from build123d import *

# Parameters (mm, degrees)
F1_DEPTH = 10.16


with BuildPart() as f1:
    # F0 (on Top) → F1 (new body)
    with BuildSketch(Plane.XY):
        with BuildLine():
            Line((-29.21, 0), (0, 0))
            Line((0, 0), (0, 8.128))
            Line((0, 8.128), (-6.604, 8.128))
            Line((-6.604, 8.128), (-6.604, 4.318))
            Line((-6.604, 4.318), (-7.62, 4.318))
            Line((-7.62, 4.318), (-7.62, 5.334))
            Line((-7.62, 5.334), (-7.62, 8.636))
            ThreePointArc((-7.62, 8.636), (-7.991974, 9.534026), (-8.89, 9.906))
            Line((-8.89, 9.906), (-26.67, 9.906))
            ThreePointArc((-26.67, 9.906), (-28.466051, 9.162051), (-29.21, 7.366))
            Line((-29.21, 7.366), (-29.21, 0))
        make_face()
    extrude(amount=F1_DEPTH)

    # F2: F1 across face


with BuildPart() as f1_1:
    add(f1.part)
    add(f1.part.mirror(Plane(origin=(0, 4.064, 5.08), x_dir=(0, 1, 0), z_dir=(1, 0, 0))))

    # F3: F1 across face


with BuildPart() as f1_2:
    add(f1_1.part)
    add(f1_1.part.mirror(Plane(origin=(0, 0, 5.08), x_dir=(1, 0, 0), z_dir=(0, -1, 0))))


solid = f1_2.part
Here's how the part is built. I have some questions about the finished solid (model axes, mm). A direction names the side the tool comes from. Give positions to 0.01 mm unless a question says otherwise; leave off trailing zeros. Order: outer loops, then holes, each group sorted by start corner. A loop starts at its lowest first (then second) coordinate and runs counter-clockwise, first axis right, second up. Notation, with made-up numbers: M -38.5,-26.75 L 9.5,-26.75 A22 ccw 9.5,-9.75 Z; hole C 77.5,29 d9. An arc over 180 degrees is marked long. Answer as a JSON object with one key per item and string values. Group by question number.
1) Please list where these lines run through material, in increasing order: L1, parallel to X at y = -7.25, z = 4.25; L2, parallel to Y at x = 5.5, z = 2.5; L3, parallel to X at y = 8.25, z = 7.25. Write a range as [from, to].
2) I'm going to push flat-ended pins straight in: pin 1 Ø0.8 at (x, z) = (7.5, 7) entering from -Y; pin 2 Ø5 at (x, z) = (1.5, 5.5) entering from +Y; pin 3 Ø1.1 at (x, z) = (-7.5, 5.5) entering from -Y. Where does each tip first touch, or does it pass through?
3) Suppose I cut it at A-A, the plane y = 5. Write out the boundary of the cut face in (x, z), plus the area to 3 significant figures.
4) On a 3-axis mill with a long thin cutter (end or side, diameter ignored), from which of +Z, -Z, +X, -X, +Y, -Y can I reach the whole of each face in a straight line? I mean faces 1 (the flat face through (0, 0, 0)), 2 (the flat face through (0, -8.128, 5)), 3 (the flat face through (7.62, 6, 5)). Say none if no direction works.
5) Suppose I cut it at C-C, the plane x = -1.5. Write out the boundary of the cut face in (y, z).
6) Suppose I cut it at B-B, the plane z = 7.75. Write out the boundary of the cut face in (x, y).
7) We'd pull the mould along X, two halves only. Please class faces 4 (the cylindrical face through (-28.45, 9.18, 5.01)), 5 (the flat face through (6.604, 6, 5)), 6 (the flat face through (29.21, 0, 5)), 7 (the flat face through (0, 0, 10.16)): pulls with the +X half, pulls with the -X half, needs draft (parallel to the pull), parting line crosses it, or undercut.
Results found:
{
 "1": {"L1": "[-29.21, -7.62], [-6.6, 6.6], [7.62, 29.21]", "L2": "[-8.13, 8.13]", "L3": "[-29.05, -7.62], [7.62, 29.05]"},
 "2": {"pin 1": "y = -9.43", "pin 2": "y = 8.13", "pin 3": "y = -9.59"},
 "3": {"outline": "M -29.21,0 L -7.62,0 L -7.62,10.16 L -29.21,10.16 Z; M -6.6,0 L 6.6,0 L 6.6,10.16 L -6.6,10.16 Z; M 7.62,0 L 29.21,0 L 29.21,10.16 L 7.62,10.16 Z", "area": "573 mm²"},
 "4": {"face 1": "-Z, +X, -X, +Y, -Y", "face 2": "+Z, -Z, -Y", "face 3": "+Z, -Z, +Y"},
 "5": {"outline": "M -8.13,0 L 8.13,0 L 8.13,10.16 L -8.13,10.16 Z"},
 "6": {"outline": "M -29.21,-7.37 A2.54 ccw -26.67,-9.91 L -8.89,-9.91 A1.27 ccw -7.62,-8.64 L -7.62,-4.32 L -6.6,-4.32 L -6.6,-8.13 L 6.6,-8.13 L 6.6,-4.32 L 7.62,-4.32 L 7.62,-8.64 A1.27 ccw 8.89,-9.91 L 26.67,-9.91 A2.54 ccw 29.21,-7.37 L 29.21,7.37 A2.54 ccw 26.67,9.91 L 8.89,9.91 A1.27 ccw 7.62,8.64 L 7.62,4.32 L 6.6,4.32 L 6.6,8.13 L -6.6,8.13 L -6.6,4.32 L -7.62,4.32 L -7.62,8.64 A1.27 ccw -8.89,9.91 L -26.67,9.91 A2.54 ccw -29.21,7.37 Z"},
 "7": {"face 4": "pulls with the -X half", "face 5": "undercut", "face 6": "pulls with the +X half", "face 7": "needs draft"}
}
